```python
from build123d import *

# Parameters (mm, degrees)
SKETCH1_R               = 1.25
BOSS_EXTRUDE1_DEPTH     = 5
BOSS_EXTRUDE2_DEPTH     = 5
FILLET2_R               = 10
CUT_EXTRUDE2_DEPTH      = 27.814458153
CUT_EXTRUDE2_DEPTH_BACK = 27.814458153
SKETCH4_W               = 2.5
SKETCH4_H               = 5
SKETCH5_W               = 2.5
SKETCH5_H               = 2.5
CUT_EXTRUDE3_DEPTH      = 1.37
FILLET3_R               = 2
SKETCH6_R               = 1.25
CUT_EXTRUDE4_DEPTH      = 27.814458153
SKETCH7_R               = 0.2
CUT_EXTRUDE5_DEPTH      = 25.573800354


with BuildPart() as part:
    # Sketch1 → Boss-Extrude1 (new body)
    with BuildSketch(Plane.XY):
        with BuildLine():
            Line((0, 2.5), (0, 5))
            Line((0, 5), (-2.5, 5))
            Line((-2.5, 5), (-2.5, 0))
            ThreePointArc((-2.5, 0), (1.767766953, -1.767766953), (0, 2.5))
        make_face()
        Circle(SKETCH1_R, mode=Mode.SUBTRACT)
    extrude(amount=BOSS_EXTRUDE1_DEPTH)

    # Sketch2 → Boss-Extrude2 (add)
    with BuildSketch(Plane.XY.offset(5)):
        with BuildLine():
            Line((-2.5, 2.5), (0, 2.5))
            ThreePointArc((0, 2.5), (-4.79077334, 13.027539424), (-7.472558856, 24.278700341))
            ThreePointArc((-7.472558856, 24.278700341), (-9.849121132, 12.279055883), (-2.5, 2.5))
        make_face()
    extrude(amount=-BOSS_EXTRUDE2_DEPTH)

    # Fillet2
    fillet2_edges = [part.edges().sort_by_distance(p)[0] for p in [
        (-2.5, 2.5, 2.5),
    ]]
    fillet(fillet2_edges, radius=FILLET2_R)

    # Sketch4 → Cut-Extrude2 (cut, two sides: drawn at the far end of the back side and taken through both)
    with BuildSketch(Plane(origin=(0, 0, 0), x_dir=(0, 0, -1), z_dir=(1, 0, 0)).offset(-CUT_EXTRUDE2_DEPTH_BACK)):
        with Locations((-2.5, 0)):
            Rectangle(SKETCH4_W, SKETCH4_H)
    extrude(amount=CUT_EXTRUDE2_DEPTH + CUT_EXTRUDE2_DEPTH_BACK, mode=Mode.SUBTRACT)

    # Sketch5 → Cut-Extrude3 (cut)
    with BuildSketch(Plane(origin=(0, 0, 0), x_dir=(0, 0, -1), z_dir=(1, 0, 0))):
        with Locations((-2.5, 3.75)):
            Rectangle(SKETCH5_W, SKETCH5_H)
    extrude(amount=-CUT_EXTRUDE3_DEPTH, mode=Mode.SUBTRACT)

    # Fillet3
    # the kernel refuses this fillet: 2 mm, written as the material it takes off along each edge
    with BuildSketch(Plane(origin=(0, 5, -4.741540982), x_dir=(0, -1, 0), z_dir=(0, 0, 1))) as fillet3_piece_1:
        with BuildLine():
            CenterArc((1.896616393, -2), FILLET3_R, 90, 71.497208819)
            Line((0, -1.365298292), (-0.037932328, -1.352604258))
            ThreePointArc((-0.037932328, -1.352604258), (-0.04, -0.682649146), (-0.04, 0))
            Line((-0.04, 0), (0, 0.04))
            Line((0, 0.04), (1.896616393, 0.04))
            Line((1.896616393, 0.04), (1.896616393, 0))
        make_face()
    extrude(amount=10.733081965, mode=Mode.SUBTRACT)
    with BuildSketch(Plane(origin=(0, 5, -0.991540982), x_dir=(-1, 0, 0), z_dir=(0, 0, 1))) as fillet3_piece_2:
        with BuildLine():
            CenterArc((2, 1.896616393), FILLET3_R, 180, 71.497208819)
            Line((0, 1.896616393), (-0.04, 1.896616393))
            Line((-0.04, 1.896616393), (-0.04, 0))
            Line((-0.04, 0), (0, -0.04))
            ThreePointArc((0, -0.04), (0.682649146, -0.04), (1.352604258, -0.037932328))
            Line((1.352604258, -0.037932328), (1.365298292, 0))
        make_face()
    extrude(amount=10.733081965, mode=Mode.SUBTRACT)

    # Sketch6 → Cut-Extrude4 (cut, through all)
    with BuildSketch(Plane(origin=(0, 0, 0), x_dir=(0, 0, -1), z_dir=(1, 0, 0))):
        with Locations((-2.5, 13)):
            Circle(SKETCH6_R)
    extrude(amount=-CUT_EXTRUDE4_DEPTH, mode=Mode.SUBTRACT)

    # Sketch7 → Cut-Extrude5 (cut, through all)
    with BuildSketch(Plane.XZ.offset(-2.5)):
        with Locations((-2.521961644, 2.5)):
            Circle(SKETCH7_R)
    extrude(amount=-CUT_EXTRUDE5_DEPTH, mode=Mode.SUBTRACT)


solid = part.part
```
The model under review builds one solid part; all positions refer to its coordinate system, in mm. A direction names the side the tool comes from. Round coordinates to 2 decimals unless told otherwise and drop trailing zeros. Loops run counter-clockwise (first coordinate to the right, second up) from the corner with the lowest first, then second, coordinate; pieces in that order, holes last. Notation, with made-up numbers: (50.5, -6.75) -> (75.5, -6.75) arc R19 ccw to (75.5, 14.25) -> close; hole circle Ø5 at (53, 56). An arc over 180 degrees is marked (long way). Answer as a JSON object with one key per item and string values. Group by question number.
1) We need section D-D on y = 11. Write out the cut boundary in (x, z), then the cut area to 3 significant figures.
2) We need section C-C on x = -5.75. Write out the cut boundary in (y, z), then the cut area to 3 significant figures.
3) For pin 1 Ø1.5 at (y, z) = (11.5, 2) entering from -X; pin 2 Ø1 at (x, z) = (-5.5, 0.5) entering from -Y; pin 3 Ø1.2 at (x, z) = (-3, 2.5) entering from -Y, all flat-tipped, find the tip position at first contact; note any pin that passes through.
4) For line 1 (Z direction, x = -7.1, y = 13); line 2 (X direction, y = 0, z = 0.85), list the stretches that pass through material, from the lowest coordinate up. Write a range as [from, to].
5) We need section B-B on x = 0.75. Write out the cut boundary in (y, z), then the cut area to 3 significant figures.
6) We need section A-A on y = 14. Write out the cut boundary in (x, z), then the cut area to 3 significant figures.
7) For faces 5 (the face through (-1, 1, 1.25)), 6 (the face through (-7.208, 11.891, 1.923)), list the 3-axis set-ups (+Z, -Z, +X, -X, +Y, -Y) from which the entire face can be reached by the end or side of a thin tool; tool diameter is ignored.
8) Mouldability with a two-part tool opening along Y and no side actions: class faces 1 (the face through (-0.27, -1.22, 4.37)), 2 (the face through (-2, 2.5, 3)), 3 (the face through (-0.37, 4.26, 0.62)), 4 (the face through (-0.27, -1.22, 0.62)) as released by +Y, released by -Y, zero draft, split by the parting line, or undercut.
Result set:
{
 "1": {"outline": "(-9.5, 0) -> (-4.05, 0) -> (-4.05, 5) -> (-9.5, 5) -> close", "area": "27.2 mm²"},
 "2": {"outline": "(4.93, 0) -> (16.09, 0) -> (16.09, 5) -> (4.93, 5) -> close; hole circle Ø2.5 at (13, 2.5)", "area": "50.9 mm²"},
 "3": {"pin 1": "x = -9.82", "pin 2": "y = 4.2", "pin 3": "y = 2.5"},
 "4": {"line 1": "[0, 1.25], [3.75, 5]", "line 2": "[-2.58, -1.25], [1.25, 2.5]"},
 "5": {"outline": "(-2.38, 0) -> (-1, 0) -> (-1, 1.25) -> (-2.38, 1.25) -> close; (-2.38, 3.75) -> (-1, 3.75) -> (-1, 5) -> (-2.38, 5) -> close; (1, 0) -> (2.38, 0) -> (2.38, 1.25) -> (1, 1.25) -> close; (1, 3.75) -> (2.38, 3.75) -> (2.38, 5) -> (1, 5) -> close", "area": "6.92 mm²"},
 "6": {"outline": "(-10.14, 0) -> (-5.12, 0) -> (-5.12, 1.75) -> (-10.14, 1.75) -> close; (-10.14, 3.25) -> (-5.12, 3.25) -> (-5.12, 5) -> (-10.14, 5) -> close", "area": "17.6 mm²"},
 "7": {"face 5": "+X, -Y", "face 6": "+X, -X"},
 "8": {"face 1": "undercut", "face 2": "released by -Y", "face 3": "released by +Y", "face 4": "undercut"}
}
